Input: dimensioned drawing with shaded views. Units: mm. Origin: part minimum x, y, z. A direction names the side the tool comes from. Coordinates: 2 decimals unless noted, no trailing zeros. Order: outer loops, then holes, each group sorted by start corner. A loop starts at its lowest first (then second) coordinate and runs counter-clockwise, first axis right, second up.
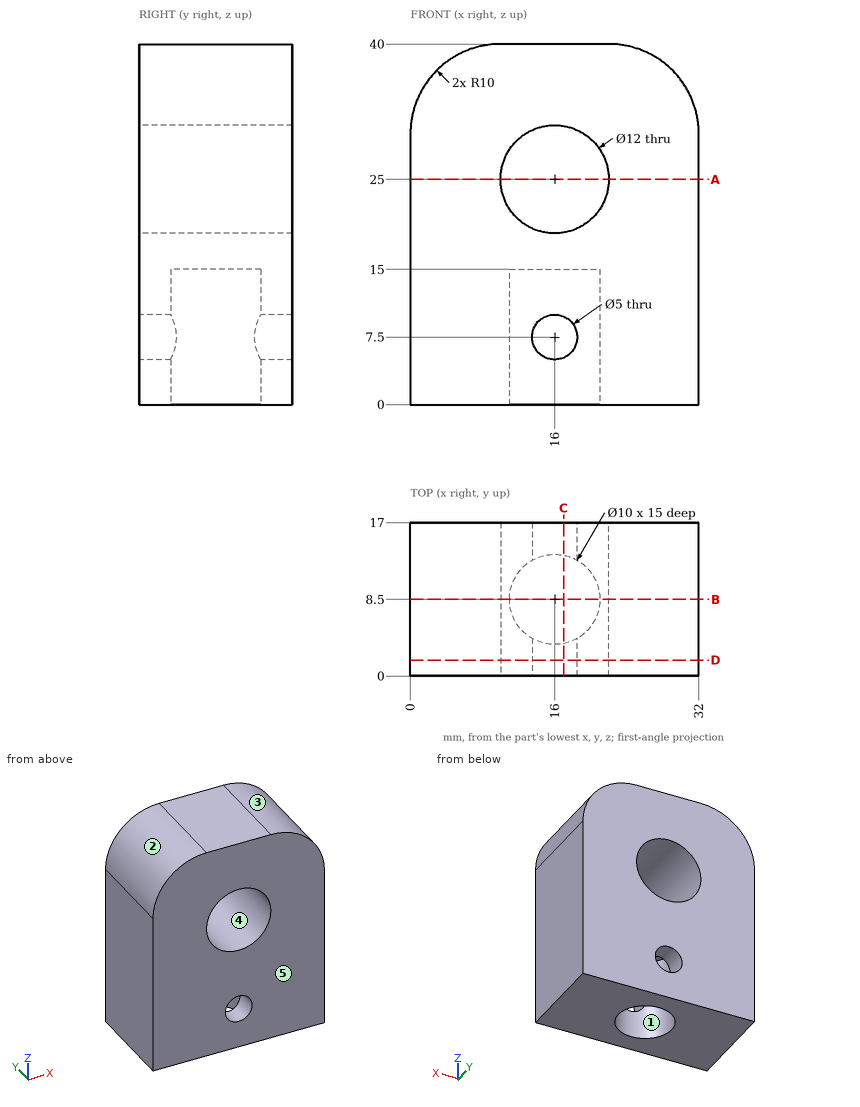
1. Pin query (flat end, axial travel): P1, Ø4, axis at x = 16, z = 7.5, coming from the +Y side. Return the tip coordinate at first contact, or that it passes through.
Findings:
P1: passes through
2. Draft query along X for the marked faces 3, 4 and 5. Return one class per face: released by +X, released by -X, zero draft, split by the parting line, or undercut.
Findings:
face 3: released by +X
face 4: undercut
face 5: zero draft
3. Section query B-B on y = 8.5. Return loops of the section in (x, z).
Findings:
outline: (0, 0) - (11, 0) - (11, 15) - (21, 15) - (21, 0) - (32, 0) - (32, 30) arc R10 ccw to (22, 40) - (10, 40) arc R10 ccw to (0, 30) - close; hole circle Ø12 at (16, 25)
4. Section query A-A on z = 25. Return loops of the section in (x, y).
Findings:
outline: (0, 0) - (10, 0) - (10, 17) - (0, 17) - close; (22, 0) - (32, 0) - (32, 17) - (22, 17) - close
5. Access query for the marked faces 1 and 2. Directions: +Z, -Z, +X, -X, +Y, -Y. A direction counts if a zero-diameter tool reaches every point of the face in a straight line with its end or side. Return the directions, or none.
Findings:
face 1: -Z
face 2: +Z, -X, +Y, -Y
6. Section query D-D on y = 1.75. Return loops of the section in (x, z).
Findings:
outline: (0, 0) - (32, 0) - (32, 30) arc R10 ccw to (22, 40) - (10, 40) arc R10 ccw to (0, 30) - close; hole circle Ø12 at (16, 25); hole circle Ø5 at (16, 7.5)
7. Ray query, line 1 (Z direction, x = 16, y = 2.45); line 2 (Z direction, x = 16, y = 12); line 3 (Z direction, x = 13.5, y = 9). Return the intervals inside material, ascending.
Findings:
line 1: z = 0 to 5, 10 to 19, 31 to 40
line 2: z = 15 to 19, 31 to 40
line 3: z = 15 to 19.55, 30.45 to 40
8. Section query C-C on x = 17. Return loops of the section in (y, z), plus the area to 3 significant figures.
Findings:
outline: (0, 0) - (3.6, 0) - (3.6, 5.21) - (0, 5.21) - close; (0, 9.79) - (3.6, 9.79) - (3.6, 15) - (13.4, 15) - (13.4, 9.79) - (17, 9.79) - (17, 19.08) - (0, 19.08) - close; (0, 30.92) - (17, 30.92) - (17, 40) - (0, 40) - close; (13.4, 0) - (17, 0) - (17, 5.21) - (13.4, 5.21) - close
area: 299 mm2
